```python
from build123d import *

# Parameters (mm, degrees)
SKETCH2_R                = 25.4
BOSS_EXTRUDE1_DEPTH      = 63.5
BOSS_EXTRUDE1_DEPTH_BACK = 17.78
SKETCH3_R                = 25.4
BOSS_EXTRUDE2_DEPTH      = 109.317536
BOSS_EXTRUDE2_TAPER      = 3.79256
SKETCH4_R                = 15.06855
CUT_EXTRUDE1_DEPTH       = 109.317536
CUT_EXTRUDE1_DRAFT       = 0.49256
SPLIT6_SURFACE_1_BACK    = 204.688
SPLIT6_SURFACE_1_DEPTH   = 409.376
CUT_EXTRUDE3_DEPTH       = 13.559536
SKETCH8_R                = 13.182228497
CUT_EXTRUDE4_DEPTH       = 13.559536


with BuildPart() as part:
    # Sketch2 → Boss-Extrude1 (new, two sides)
    with BuildSketch(Plane(origin=(0, 0, 0), x_dir=(1, 0, 0), z_dir=(0, 1, 0))) as boss_extrude1_sk:
        with Locations(Location((0, 0, 0), (0, 0, 270))):
            Circle(SKETCH2_R)
    extrude(amount=BOSS_EXTRUDE1_DEPTH)
    extrude(boss_extrude1_sk.sketch, amount=-BOSS_EXTRUDE1_DEPTH_BACK)

    # Sketch3 → Boss-Extrude2 (add)
    with BuildSketch(Plane(origin=(0, 63.5, 0), x_dir=(1, 0, 0), z_dir=(0, 1, 0))):
        with Locations(Location((0, 0, 0), (0, 0, 270))):
            Circle(SKETCH3_R)
    extrude(amount=BOSS_EXTRUDE2_DEPTH, taper=BOSS_EXTRUDE2_TAPER)


with BuildPart() as cut_extrude1_tool:
    # Sketch4 → Cut-Extrude1 (with draft: the straight prism first)
    with BuildSketch(Plane(origin=(0, 172.817536, 0), x_dir=(1, 0, 0), z_dir=(0, 1, 0))):
        Circle(SKETCH4_R)
    extrude(amount=-CUT_EXTRUDE1_DEPTH)
    # Cut-Extrude1: the draft: its side faces are tilted about the plane it starts from
    cut_extrude1_sides = [cut_extrude1_tool.faces().sort_by_distance(p)[0] for p in [
        (-15.06855, 118.158768, 0),
    ]]
    draft(cut_extrude1_sides, Plane(origin=(0, 172.817536, 0), x_dir=(1, 0, 0), z_dir=(0, 1, 0)), CUT_EXTRUDE1_DRAFT)


with BuildPart() as part_1:
    add(part.part)

    # Cut-Extrude1: cut by cut_extrude1_tool
    add(cut_extrude1_tool.part, mode=Mode.SUBTRACT)

    # Split6: cut with a surface, the side behind it stays
    # Split6 surface: a surface, the sketch's curves swept straight by 409.376 mm
    with BuildLine(Plane(origin=(0, 0, 0), x_dir=(1, 0, 0), z_dir=(0, 1, 0)).offset(-SPLIT6_SURFACE_1_BACK), mode=Mode.PRIVATE) as split6_surface_1_path:
        Line((0, 25.4), (0, -25.4))
    split6_surface_1 = Shell.extrude(split6_surface_1_path.wire(), (0 * SPLIT6_SURFACE_1_DEPTH, 1 * SPLIT6_SURFACE_1_DEPTH, 0 * SPLIT6_SURFACE_1_DEPTH))
    split(bisect_by=split6_surface_1, keep=Keep.BOTTOM)

    # Sketch7 → Cut-Extrude3 (cut)
    with BuildSketch(Plane(origin=(0, 0, 0), x_dir=(0, 0, -1), z_dir=(1, 0, 0))):
        Polygon((-20.392899445, 0), (-20.392899445, 50.791761633), (20.25247775, 50.791761633), (20.25247775, -12.77676991), (-20.392899445, -12.77676991), align=None)
    extrude(amount=-CUT_EXTRUDE3_DEPTH, mode=Mode.SUBTRACT)

    # Sketch8 → Cut-Extrude4 (cut)
    with BuildSketch(Plane(origin=(0, 63.5, 0), x_dir=(1, 0, 0), z_dir=(0, 1, 0))):
        Circle(SKETCH8_R)
    extrude(amount=-CUT_EXTRUDE4_DEPTH, mode=Mode.SUBTRACT)


solid = part_1.part
```
Source: CAD feature listing. Evaluate the final solid. Frame: model axes, mm. A direction names the side the tool comes from. Give positions to 0.01 mm unless a question says otherwise; leave off trailing zeros. Loops run counter-clockwise (first coordinate to the right, second up) from the corner with the lowest first, then second, coordinate; pieces in that order, holes last. Notation, with made-up numbers: M -23,-12.5 L 22,-12.5 A22 cw 22,20.5 Z; hole C 26,46.5 d2. An arc over 180 degrees is marked long. Put each result on its own line as item: value.
Q1. Line query: probe 1 along Y at (x, z) = (-5.5, 13.5); probe 2 along Y at (x, z) = (-7, 4.5); probe 3 along Z at (x, y) = (-1.5, 94). Output: solid intervals per line, ascending. Write a range as [from, to].
Response values:
probe 1: y = [-17.78, -12.78], [50.79, 63.5]
probe 2: y = [-17.78, -12.78]
probe 3: z = [-23.33, -15.67], [15.67, 23.33]
Q2. Section B-B (y = 126.5). Return the cut outline in (x, z).
Response values:
outline: M 0,-21.22 L 0,-15.47 A15.47 cw 0,15.47 L 0,21.22 A21.22 ccw Z
Q3. Mould query, pull axis Z, two halves, no side actions, for faces 4 (the flat face through (-7, -12.777, 0)), 5 (the flat face through (0, 56, -15)), 6 (the conical face through (-21.72, 118.92, -0.48)). Classes: released by +Z, released by -Z, zero draft, split by the parting line, or undercut.
Response values:
face 4: undercut
face 5: zero draft
face 6: split by the parting line
Q4. Section C-C (y = 70.5). Return the cut outline in (x, z).
Response values:
outline: M 0,-24.94 L 0,-15.95 A15.95 cw 0,15.95 L 0,24.94 A24.94 ccw Z
Q5. Pin query (flat end, axial travel): P1, Ø6, axis at x = -9.5, y = 106, coming from the +Z side; P2, Ø6, axis at x = -10.5, y = 7, coming from the +Z side; P3, Ø6, axis at y = 37, z = 0.5, coming from the -X side; P4, Ø15, axis at x = -4, y = 28.5, coming from the +Z side. Return the tip coordinate at first contact, or that it passes through.
Response values:
P1: stops at z = 21.65
P2: stops at z = 24.27
P3: stops at x = -25.4
P4: stops at z = 25.4
Q6. Section A-A (y = 49). Return the cut outline in (x, z), and give its area (3 significant figures).
Response values:
outline: M -13.56,-20.25 L -13.56,20.39 L 0,20.39 L 0,25.4 A25.4 ccw 0,-25.4 L 0,-20.25 Z
area: 462 mm²
Q7. Reachability of faces 1 (the cylindrical face through (-25.394, 23.429, -0.559)), 2 (the cylindrical face through (-13.18, 57.23, -0.29)), 3 (the flat face through (-7, 19, 20.393)) from +Z, -Z, +X, -X, +Y, -Y: full face, straight path, thin tool, end or side. Return the list, or none.
Response values:
face 1: -X, +Y, -Y
face 2: +X, +Y
face 3: +X
